Check sheet for the drawn part. Datum: minimum x, y, z corner. Units: mm. Give positions to 0.01 mm unless a question says otherwise; leave off trailing zeros. Loops run counter-clockwise (first coordinate to the right, second up) from the corner with the lowest first, then second, coordinate; pieces in that order, holes last. Notation, with made-up numbers: (-20, 48.25) - (-3, 48.25) arc R30 cw to (-3, 83.25) - close; hole circle Ø6 at (19.5, 68). An arc over 180 degrees is marked (long way). Use one line per item in the form item = value.
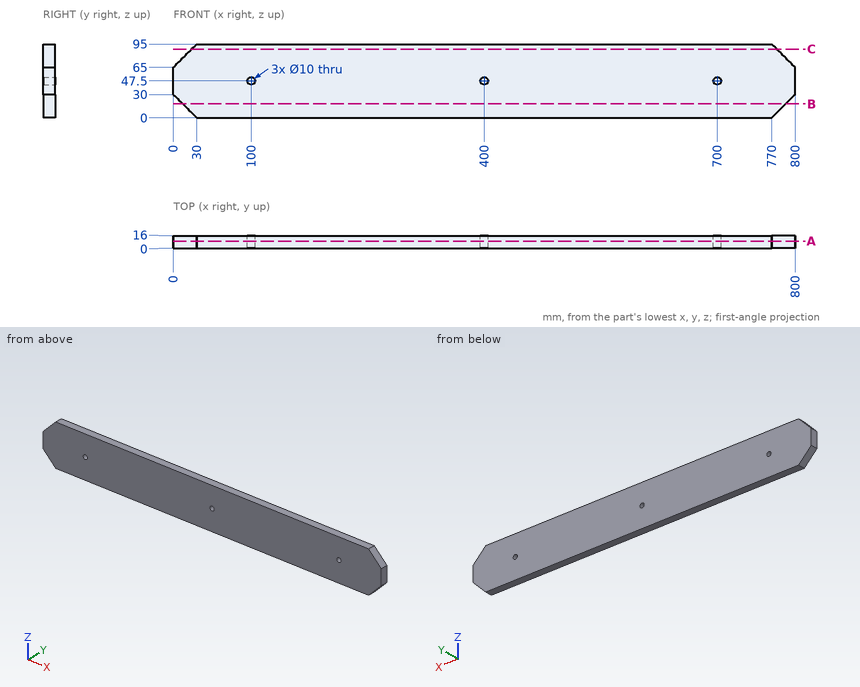
Item 1: Section check B-B on z = 18. Record the boundary of the cut face in (x, y).
Answer block:
outline = (12, 0) - (788, 0) - (788, 16) - (12, 16) - close
Item 2: Thickness scan on L1, parallel to Z at x = 400, y = 11.75; L2, parallel to X at y = 13, z = 5; L3, parallel to X at y = 4.5, z = 29. Record the ranges inside material, lowest first.
Answer block:
L1 = 0 to 42.5, 52.5 to 95
L2 = 25 to 775
L3 = 1 to 799
Item 3: Gauge pin test, flat end, axial feed: P1, Ø9, axis at x = 400, z = 47.5, coming from the -Y side. Record the tip position at first contact, or that the pin passes through.
Answer block:
P1 = through
Item 4: Section check C-C on z = 88.5. Record the boundary of the cut face in (x, y).
Answer block:
outline = (23.5, 0) - (776.5, 0) - (776.5, 16) - (23.5, 16) - close
Item 5: Section check A-A on y = 9. Record the boundary of the cut face in (x, z).
Answer block:
outline = (0, 30) - (30, 0) - (770, 0) - (800, 30) - (800, 65) - (770, 95) - (30, 95) - (0, 65) - close; hole circle Ø10 at (100, 47.5); hole circle Ø10 at (400, 47.5); hole circle Ø10 at (700, 47.5)
